Source: three-view drawing plus pictorial views. Frame: mm from the lowest corner of the part. A direction names the side the tool comes from. Round coordinates to 2 decimals unless told otherwise and drop trailing zeros. Write each loop counter-clockwise with the first axis right and the second up, starting at its lowest first coordinate (ties: lowest second). Pieces come first, ordered by that corner, then holes.
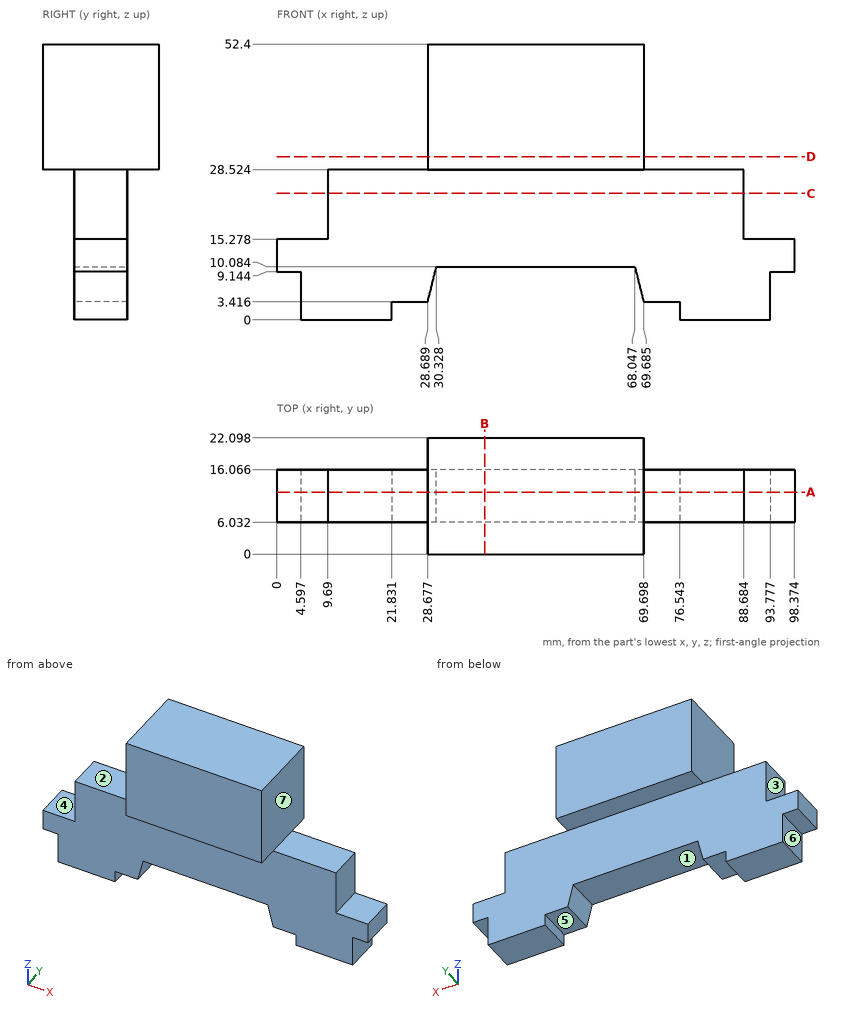
1) Section C-C on z = 24. Output: boundary loops of the cut face in (x, y) (1 decimal).
2) Section A-A on y = 11.75. Output: boundary loops of the cut face in (x, z) (1 decimal).
3) Section D-D on z = 31. Output: boundary loops of the cut face in (x, y).
4) Reachability of the marked faces 4, 5, 6 and 7 from +Z, -Z, +X, -X, +Y, -Y: full face, straight path, thin tool, end or side. Return the list, or none.
5) Draft query along X for the marked faces 1, 2 and 3. Return one class per face: pulls with the +X half, pulls with the -X half, needs draft (parallel to the pull), parting line crosses it, or undercut.
6) Line query: probe 1 along X at (y, z) = (10.75, 10) (1 decimal); probe 2 along X at (y, z) = (11.5, 3.5) (1 decimal); probe 3 along Y at (x, z) = (70, 24) (1 decimal). Output: solid intervals per line, ascending.
7) Section B-B on x = 39.5. Output: boundary loops of the cut face in (y, z) (1 decimal).
8) First-contact query: P1, Ø3, axis at x = 15, y = 8.5, coming from the +Z side; P2, Ø1.5, axis at y = 11, z = 6.5, coming from the +X side; P3, Ø6, axis at x = 62, z = 20.5, coming from the +Y side (1 decimal); P4, Ø5, axis at x = 41, z = 6, coming from the -Y side. Flat tips, straight axial feed; report the tip coordinate or a pass-through.
Filled in:
1. outline: (9.7, 6) - (88.7, 6) - (88.7, 16.1) - (9.7, 16.1) - close
2. outline: (0, 9.1) - (4.6, 9.1) - (4.6, 0) - (21.8, 0) - (21.8, 3.4) - (28.7, 3.4) - (30.3, 10.1) - (68, 10.1) - (69.7, 3.4) - (76.5, 3.4) - (76.5, 0) - (93.8, 0) - (93.8, 9.1) - (98.4, 9.1) - (98.4, 15.3) - (88.7, 15.3) - (88.7, 28.5) - (69.7, 28.5) - (69.7, 52.4) - (28.7, 52.4) - (28.7, 28.5) - (9.7, 28.5) - (9.7, 15.3) - (0, 15.3) - close
3. outline: (28.68, 0) - (69.7, 0) - (69.7, 22.1) - (28.68, 22.1) - close
4. face 4: +Z, -X, +Y, -Y
4. face 5: -Z, +Y, -Y
4. face 6: -Z, -X, +Y, -Y
4. face 7: +Z, +X, +Y, -Y
5. face 1: undercut
5. face 2: needs draft
5. face 3: pulls with the -X half
6. probe 1: x = 0 to 30.3, 68.1 to 98.4
6. probe 2: x = 4.6 to 28.7, 69.7 to 93.8
6. probe 3: y = 6 to 16.1
7. outline: (0, 28.5) - (6, 28.5) - (6, 10.1) - (16.1, 10.1) - (16.1, 28.5) - (22.1, 28.5) - (22.1, 52.4) - (0, 52.4) - close
8. P1: stops at z = 28.52
8. P2: stops at x = 93.78
8. P3: stops at y = 16.1
8. P4: passes through
